Verification items for the finished model (mm, model axes). Give positions to 0.01 mm unless a question says otherwise; leave off trailing zeros. Order: outer loops, then holes, each group sorted by start corner. A loop starts at its lowest first (then second) coordinate and runs counter-clockwise, first axis right, second up. Notation, with made-up numbers: (-25.75, 0.5) -> (23.25, 0.5) arc R21 cw to (23.25, 13.5) -> close; hole circle Ø8 at (31.5, 22.25). An arc over 180 degrees is marked (long way). Write each question's results on one line, items separated by ' | '. Start each with the question number.
1. Cross-section at C-C, the plane z = 23. Enter the section's corners in (x, y), then the cut area to 3 significant figures.
2. Cross-section at A-A, the plane y = 7.75. Enter the section's corners in (x, z).
3. Depth check by flat-ended pin: pin 1 Ø4 at (y, z) = (0, 207.8) entering from +X. Enter the tip coordinate at first touch or a pass-through.
4. Cross-section at B-B, the plane z = 200. Enter the section's corners in (x, y), then the cut area to 3 significant figures.
5. Material ranges on L1, parallel to Z at x = -12.25, y = 0; L2, parallel to Z at x = 11.9, y = -2.7; L3, parallel to X at y = 11.1, z = 200, recorded low to high. Write a range as from..to.
from build123d import *

# Parameters (mm, degrees)
SKETCH_1_W          = 25.4
SKETCH_1_H          = 25.4
EXTRUDE_1_DEPTH     = 250
SKETCH_1_3_W        = 21.4
SKETCH_1_3_H        = 21.4
CUT_EXTRUDE_1_DEPTH = 251.644329679
SKETCH_2_R          = 2.15
CUT_EXTRUDE_2_DEPTH = 3
SKETCH_3_R          = 2.15
CUT_EXTRUDE_3_DEPTH = 3
SKETCH_4_R          = 2.15
CUT_EXTRUDE_4_DEPTH = 3
SKETCH_5_R          = 2.150000004
CUT_EXTRUDE_5_DEPTH = 3
SKETCH_6_R          = 2.5
CUT_EXTRUDE_6_DEPTH = 10
SKETCH_7_R          = 2.5
CUT_EXTRUDE_7_DEPTH = 10
SKETCH_9_R          = 2
CUT_EXTRUDE_8_DEPTH = 25.4
SKETCH_10_R         = 2
CUT_EXTRUDE_9_DEPTH = 25.4


with BuildPart() as part:
    # Sketch 1 → Extrude 1 (new body)
    with BuildSketch(Plane.XY):
        Rectangle(SKETCH_1_W, SKETCH_1_H)
    extrude(amount=EXTRUDE_1_DEPTH)

    # Sketch 1_3 → Cut-Extrude 1 (cut, through all)
    with BuildSketch(Plane.XY):
        Rectangle(SKETCH_1_3_W, SKETCH_1_3_H)
    extrude(amount=CUT_EXTRUDE_1_DEPTH, mode=Mode.SUBTRACT)

    # Sketch 2 → Cut-Extrude 2 (cut)
    with BuildSketch(Plane(origin=(12.7, 0, 0), x_dir=(0, 0, -1), z_dir=(1, 0, 0))):
        with Locations(Location((-232.3, 0, 0), (0, 0, 90))):
            Circle(SKETCH_2_R)
        with Locations(Location((-207.8, 0, 0), (0, 0, 90))):
            Circle(SKETCH_2_R)
    extrude(amount=-CUT_EXTRUDE_2_DEPTH, mode=Mode.SUBTRACT)

    # Sketch 3 → Cut-Extrude 3 (cut)
    with BuildSketch(Plane.XZ.offset(12.7)):
        with Locations(Location((0, 232.3, 0), (0, 0, 270))):
            Circle(SKETCH_3_R)
        with Locations(Location((0, 207.8, 0), (0, 0, 270))):
            Circle(SKETCH_3_R)
    extrude(amount=-CUT_EXTRUDE_3_DEPTH, mode=Mode.SUBTRACT)

    # Sketch 4 → Cut-Extrude 4 (cut)
    with BuildSketch(Plane(origin=(12.7, 0, 0), x_dir=(0, 0, -1), z_dir=(1, 0, 0))):
        with Locations(Location((-42.199999985, -1e-08, 0), (0, 0, 90))):
            Circle(SKETCH_4_R)
        with Locations(Location((-17.699999985, -1e-08, 0), (0, 0, 90))):
            Circle(SKETCH_4_R)
    extrude(amount=-CUT_EXTRUDE_4_DEPTH, mode=Mode.SUBTRACT)

    # Sketch 5 → Cut-Extrude 5 (cut)
    with BuildSketch(Plane.XZ.offset(12.7)):
        with Locations(Location((0, 42.199999986, 0), (0, 0, 270))):
            Circle(SKETCH_5_R)
        with Locations(Location((0, 17.699999986, 0), (0, 0, 270))):
            Circle(SKETCH_5_R)
    extrude(amount=-CUT_EXTRUDE_5_DEPTH, mode=Mode.SUBTRACT)

    # Sketch 6 → Cut-Extrude 6 (cut)
    with BuildSketch(Plane.ZY.offset(12.7)):
        with Locations(Location((100, 0, 0), (0, 0, 270))):
            Circle(SKETCH_6_R)
        with Locations(Location((150, 0, 0), (0, 0, 270))):
            Circle(SKETCH_6_R)
        with Locations(Location((200, 0, 0), (0, 0, 270))):
            Circle(SKETCH_6_R)
        with Locations(Location((50, 0, 0), (0, 0, 270))):
            Circle(SKETCH_6_R)
    extrude(amount=-CUT_EXTRUDE_6_DEPTH, mode=Mode.SUBTRACT)

    # Sketch 7 → Cut-Extrude 7 (cut)
    with BuildSketch(Plane(origin=(0, 12.7, 0), x_dir=(1, 0, 0), z_dir=(0, 1, 0))):
        with Locations(Location((0, -50, 0), (0, 0, 270))):
            Circle(SKETCH_7_R)
        with Locations(Location((0, -100, 0), (0, 0, 270))):
            Circle(SKETCH_7_R)
        with Locations(Location((0, -150, 0), (0, 0, 270))):
            Circle(SKETCH_7_R)
        with Locations(Location((0, -200, 0), (0, 0, 270))):
            Circle(SKETCH_7_R)
    extrude(amount=-CUT_EXTRUDE_7_DEPTH, mode=Mode.SUBTRACT)

    # Sketch 9 → Cut-Extrude 8 (cut)
    with BuildSketch(Plane.XZ.offset(12.7)):
        with Locations(Location((2.7, 165, 0), (0, 0, 270))):
            Circle(SKETCH_9_R)
        with Locations(Location((2.7, 85, 0), (0, 0, 270))):
            Circle(SKETCH_9_R)
    extrude(amount=-CUT_EXTRUDE_8_DEPTH, mode=Mode.SUBTRACT)

    # Sketch 10 → Cut-Extrude 9 (cut)
    with BuildSketch(Plane(origin=(12.7, 0, 0), x_dir=(0, 0, -1), z_dir=(1, 0, 0))):
        with Locations(Location((-85, -2.7, 0), (0, 0, 90))):
            Circle(SKETCH_10_R)
        with Locations(Location((-165, -2.7, 0), (0, 0, 90))):
            Circle(SKETCH_10_R)
    extrude(amount=-CUT_EXTRUDE_9_DEPTH, mode=Mode.SUBTRACT)


solid = part.part
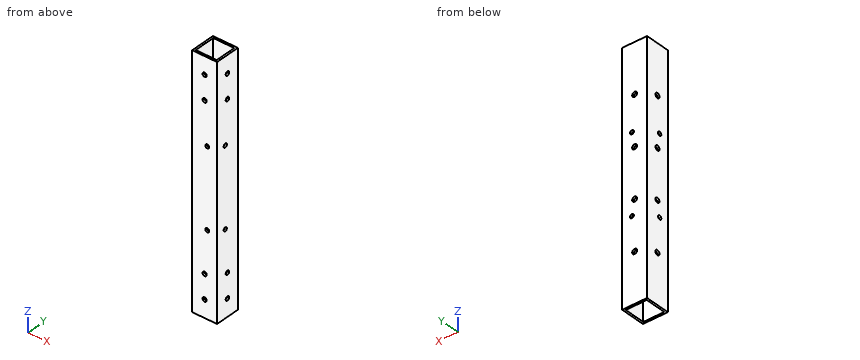
Results below:
1) outline: (-12.7, -12.7) -> (12.7, -12.7) -> (12.7, 12.7) -> (-12.7, 12.7) -> close; hole (-10.7, -10.7) -> (10.7, -10.7) -> (10.7, 10.7) -> (-10.7, 10.7) -> close | area: 187 mm²
2) outline: (-12.7, 0) -> (-10.7, 0) -> (-10.7, 250) -> (-12.7, 250) -> close; (10.7, 0) -> (12.7, 0) -> (12.7, 250) -> (10.7, 250) -> close
3) pin 1: stops at x = -10.7
4) outline: (-12.7, -12.7) -> (12.7, -12.7) -> (12.7, 12.7) -> (2.5, 12.7) -> (2.5, 10.7) -> (10.7, 10.7) -> (10.7, -10.7) -> (-10.7, -10.7) -> (-10.7, -2.5) -> (-12.7, -2.5) -> close; (-12.7, 2.5) -> (-10.7, 2.5) -> (-10.7, 10.7) -> (-2.5, 10.7) -> (-2.5, 12.7) -> (-12.7, 12.7) -> close | area: 167 mm²
5) L1: z = 0..47.5, 52.5..97.5, 102.5..147.5, 152.5..197.5, 202.5..250 | L2: z = 0..83, 87..163, 167..250 | L3: x = -12.7..-2.5, 2.5..12.7
